Build history of the part. All positions in model axes, mm. Round coordinates to 2 decimals unless told otherwise and drop trailing zeros. Order: outer loops, then holes, each group sorted by start corner. A loop starts at its lowest first (then second) coordinate and runs counter-clockwise, first axis right, second up. Notation, with made-up numbers: (86.5, 16.5) -> (96.5, 16.5) arc R13 cw to (96.5, 24.5) -> close; hole circle Ø4 at (23, 42.25). An arc over 180 degrees is marked (long way). Use a Markdown table: item, result. Add a question column.
Item 1: Slice it at A-A, the plane y = -5. Give the cut face in (x, z).
Item 2: Pin check, flat tips, straight feed: pin 1 (3.5 mm diameter, centred on x = 5, z = 16, fed in from +Y); pin 2 (1.5 mm diameter, centred on y = -7, z = 13.5, fed in from -X). Stop position of each tip, or through.
Item 3: Two-plate mould, pull along Z, no slides. Class faces 1 (the face through (4.54, -4.93, 34.05)), 2 (the face through (5, -5, 0)), 3 (the face through (5, -5, 48)): released by +Z, released by -Z, zero draft, split by the parting line, or undercut.
Item 4: Probe L1, parallel to Y at x = 6.5, z = 8; L2, parallel to Z at x = 4, y = -4.25; L3, parallel to Z at x = 5, y = -2. List the from-to ranges inside material, lowest first.
Item 5: Slice it at D-D, the plane x = 9. Give the cut face in (y, z).
Item 6: Slice it at B-B, the plane x = 5. Give the cut face in (y, z), plus the area to 3 significant figures.
Item 7: Slice it at C-C, the plane z = 32. Give the cut face in (x, y), plus the area to 3 significant figures.
from build123d import *

# Parameters (mm, degrees)
SKETCH_1_W          = 10
SKETCH_1_H          = 10
EXTRUDE_1_DEPTH     = 48
SKETCH_2_R          = 2.1
CUT_EXTRUDE_1_DEPTH = 48
SKETCH_3_R          = 2.1
CUT_EXTRUDE_2_DEPTH = 48


with BuildPart() as part:
    # 草图1 → 凸台-拉伸1 (new body)
    with BuildSketch(Plane.XY):
        with Locations((5, -5)):
            Rectangle(SKETCH_1_W, SKETCH_1_H)
    extrude(amount=EXTRUDE_1_DEPTH)

    # 草图2 → 切除-拉伸1 (cut)
    with BuildSketch(Plane(origin=(10, 0, 0), x_dir=(0, 0, -1), z_dir=(1, 0, 0))):
        with Locations((-40, -5)):
            Circle(SKETCH_2_R)
        with Locations((-8, -5)):
            Circle(SKETCH_2_R)
    extrude(amount=-CUT_EXTRUDE_1_DEPTH, mode=Mode.SUBTRACT)

    # 草图3 → 切除-拉伸2 (cut)
    with BuildSketch(Plane(origin=(0, 0, 0), x_dir=(1, 0, 0), z_dir=(0, 1, 0))):
        with Locations((5, -16)):
            Circle(SKETCH_3_R)
        with Locations((5, -32)):
            Circle(SKETCH_3_R)
    extrude(amount=-CUT_EXTRUDE_2_DEPTH, mode=Mode.SUBTRACT)


solid = part.part
Check sheet entries:
| question | item | result |
|---|---|---|
| 1 | outline | (0, 0) -> (10, 0) -> (10, 5.9) -> (0, 5.9) -> close; (0, 10.1) -> (10, 10.1) -> (10, 37.9) -> (0, 37.9) -> close; (0, 42.1) -> (10, 42.1) -> (10, 48) -> (0, 48) -> close; hole circle Ø4.2 at (5, 16); hole circle Ø4.2 at (5, 32) |
| 2 | pin 1 | through |
| 2 | pin 2 | x = 0 |
| 3 | face 1 | undercut |
| 3 | face 2 | released by -Z |
| 3 | face 3 | released by +Z |
| 4 | L1 | -10 to -7.1, -2.9 to 0 |
| 4 | L2 | 0 to 6.04, 9.96 to 14.15, 17.85 to 30.15, 33.85 to 38.04, 41.96 to 48 |
| 4 | L3 | 0 to 13.9, 18.1 to 29.9, 34.1 to 48 |
| 5 | outline | (-10, 0) -> (0, 0) -> (0, 48) -> (-10, 48) -> close; hole circle Ø4.2 at (-5, 8); hole circle Ø4.2 at (-5, 40) |
| 6 | outline | (-10, 0) -> (0, 0) -> (0, 13.9) -> (-10, 13.9) -> close; (-10, 18.1) -> (0, 18.1) -> (0, 29.9) -> (-10, 29.9) -> close; (-10, 34.1) -> (0, 34.1) -> (0, 48) -> (-10, 48) -> close; hole circle Ø4.2 at (-5, 8); hole circle Ø4.2 at (-5, 40) |
| 6 | area | 368 mm2 |
| 7 | outline | (0, -10) -> (2.9, -10) -> (2.9, 0) -> (0, 0) -> close; (7.1, -10) -> (10, -10) -> (10, 0) -> (7.1, 0) -> close |
| 7 | area | 58.0 mm2 |
